Autodesk Inventor part; units mm, degrees
ref_plane "YZ Plane" through (0, 0, 0) normal (1, 0, 0) x (0, 1, 0)
ref_plane "XZ Plane" through (0, 0, 0) normal (0, 1, 0) x (-1, 0, 0)
ref_plane "XY Plane" through (0, 0, 0) normal (0, 0, 1) x (1, 0, 0)
sketch "Sketch13" plane through (0, 0, 0) normal (0, 1, 0) x (-1, 0, 0)
  line L0 (0, 0) -> (112, 0)
  line L1 (112, 0) -> (112, 40)
  line L2 (112, 40) -> (0, 40)
  line L3 (0, 40) -> (0, 0)
  dimension "d51" = 112
  dimension "d52" = 40
extrude "Extrusion11" add sketch "Sketch13" along normal blind 40
sketch "Sketch14" plane through (-112, 0, 40) normal (0, 0, 1) x (1, 0, 0)
  line L0 (0, 0) -> (0, 40)
  arc A0 (88.2072, 0) -> (23.7928, 0) centre (56, 0) ccw
  line L1 (23.7928, 0) -> (88.2072, 0)
  dimension "d88" = 32.2072
extrude "Extrusion12" cut sketch "Sketch14" against normal blind 40
sketch "Sketch15" plane through (0, 0, 0) normal (0, -1, 0) x (1, 0, 0)
  line L0 (-88.2072, 0) -> (-88.2072, 40)
  line L1 (-112, 40) -> (-88.2072, 40)
  line L2 (-112, 0) -> (-112, 40)
  line L3 (-88.2072, 0) -> (-112, 0)
  line L4 (-100.1315, 0) -> (-100.1315, 2.5) construction
  line L5 (-101.9977, 40) -> (-101.9977, 37.5) construction
  line L6 (-112, 20) -> (-109, 20) construction
  line L7 (-88.2072, 20) -> (-94.2072, 20) construction
  line L8 (-109, 37.5) -> (-96, 37.5)
  line L9 (-96, 37.5) -> (-96, 2.5)
  line L10 (-96, 2.5) -> (-109, 2.5)
  line L11 (-109, 2.5) -> (-109, 37.5)
  line L12 (-23.7928, 40) -> (-23.7928, 0)
  line L13 (-23.7928, 40) -> (-23.7928, 0)
  line L14 (0, 0) -> (-23.7928, 0)
  line L15 (0, 40) -> (0, 0)
  line L16 (-23.7928, 40) -> (0, 40)
  line L17 (0, 20) -> (-3, 20) construction
  line L18 (-11.8964, 0) -> (-11.8964, 2.5) construction
  line L19 (-11.8964, 40) -> (-11.8964, 37.5) construction
  line L20 (-23.7928, 20) -> (-17.7928, 20) construction
  line L21 (-16, 37.5) -> (-3, 37.5)
  line L22 (-3, 37.5) -> (-3, 2.5)
  line L23 (-3, 2.5) -> (-16, 2.5)
  line L24 (-16, 2.5) -> (-16, 37.5)
  dimension "d60" = 2.5
  dimension "d62" = 2.5
  dimension "d63" = 3
  dimension "d64" = 6
  dimension "d65" = 3
  dimension "d66" = 2.5
  dimension "d67" = 2.5
  dimension "d68" = 6
extrude "Extrusion13" cut sketch "Sketch15" against normal blind 30 contours L8 L9 L10 L11 | L21 L22 L23 L24
sketch "Sketch16" plane through (0, 30, 0) normal (0, -1, 0) x (1, 0, 0)
  line L0 (-16, 37.5) -> (-3, 37.5)
  line L1 (-16, 2.5) -> (-16, 37.5)
  line L2 (-3, 2.5) -> (-16, 2.5)
  line L3 (-3, 37.5) -> (-3, 2.5)
  circle A0 centre (-102.5, 20) radius 9
  circle A1 centre (-9.5, 20) radius 9
  point P0 (0, 0)
  dimension "d71" = 18
  dimension "d72" = 18
extrude "Extrusion14" add sketch "Sketch16" along normal blind 30 contours A1 L3 L1 | L1 A1 | A1 L3 | A0
sketch "Sketch17" plane through (0, 0, 0) normal (0, -1, 0) x (1, 0, 0)
  arc A0 (-109, 13.7751) -> (-96, 13.7751) centre (-102.5, 20) ccw
  line L0 (-16, 26.2249) -> (-16, 37.5)
  line L1 (-16, 37.5) -> (-3, 37.5)
  line L2 (-3, 37.5) -> (-3, 26.2249)
  arc A1 (-3, 26.2249) -> (-16, 26.2249) centre (-9.5, 20) ccw
  line L3 (-23.7928, 40) -> (-23.7928, 0)
  line L4 (0, 0) -> (-23.7928, 0)
  line L5 (0, 40) -> (0, 0)
  line L6 (-23.7928, 40) -> (0, 40)
  arc A2 (-16, 13.7751) -> (-3, 13.7751) centre (-9.5, 20) ccw
  line L7 (-3, 13.7751) -> (-3, 2.5)
  line L8 (-3, 2.5) -> (-16, 2.5)
  line L9 (-16, 2.5) -> (-16, 13.7751)
  circle A3 centre (-102.5, 20) radius 5.5
  circle A4 centre (-9.5, 20) radius 5.5
  dimension "d75" = 11
  dimension "d76" = 11
extrude "Extrusion15" cut sketch "Sketch17" against normal blind 76.2 contours A3 | A4
sketch "Sketch18" plane through (0, 40, 0) normal (0, 1, 0) x (1, 0, 0)
  circle A0 centre (-102.5, -20) radius 5.5
  circle A1 centre (-9.5, -20) radius 5.5
  circle A2 centre (-102.5, -20) radius 9
  circle A3 centre (-9.5, -20) radius 9
  dimension "d79" = 18
  dimension "d81" = 18
extrude "Extrusion16" cut sketch "Sketch18" against normal blind 8
fillet "Fillet3" radius 3.175 6 edges at (-16, 15, 2.5) (-3, 15, 2.5) (-16, 15, 37.5) (-3, 15, 37.5) (0, 20, 40) (0, 20, 0)
fillet "Fillet4" radius 3.175 6 edges at (-112, 20, 0) (-112, 20, 40) (-109, 15, 37.5) (-109, 15, 2.5) (-96, 15, 2.5) (-96, 15, 37.5)
fillet "Fillet5" radius 1 8 edges at (-0.9299, 40, 39.0701) (0, 40, 20) (-0.9299, 40, 0.9299) (-56, 40, 0) (-111.0701, 40, 0.9299) (-112, 40, 20) (-111.0701, 40, 39.0701) (-56, 40, 40)
equation "\"d62\" = d60"
equation "\"d65\" = d63"
equation "\"d66\" = d60"
equation "\"d67\" = d66"
equation "\"d68\" = d64"
equation "\"d81\" = d79"
properties part number "2.5 CIM mount" material "ABS Plastic"
Input: part model. Units: mm. Frame: model coordinates. A direction names the side the tool comes from. Coordinates: 2 decimals unless noted, no trailing zeros. Loops run counter-clockwise (first coordinate to the right, second up) from the corner with the lowest first, then second, coordinate; pieces in that order, holes last. Notation, with made-up numbers: (-14, 35.5) -> (-4, 35.5) arc R12 cw to (-4, 52.5) -> close; hole circle Ø3 at (-7, 34.25). An arc over 180 degrees is marked (long way). Write each question's results on one line, items separated by ' | '. Start each with the question number.
Q1. Section D-D, the plane x = -56. Return the cut outline in (y, z), plus the area to 3 significant figures.
Q2. Section C-C, the plane y = 25.5. State how many separate pieces and enclosed holes the cut face has, plus the area to 3 significant figures.
Q3. Section A-A, the plane x = -102.5. Return the cut outline in (y, z).
Q4. Pull-direction query (Z, two-part tool) for faces 4 (the cylindrical face through (-55.3, 32.2, 20.3)), 5 (the cylindrical face through (-3.95, 15.21, 36.59)), 6 (the flat face through (-109, 15, 10)), 7 (the flat face through (-57, 37, 40)); classes: released by +Z, released by -Z, zero draft, split by the parting line, or undercut.
Q5. Pin query (flat end, axial travel): pin 1 (8 mm diameter, centred on x = -45.5, z = 16, fed in from -Y); pin 2 (10 mm diameter, centred on x = -65.5, y = 20.5, fed in from -Z); pin 3 (10 mm diameter, centred on x = -44.5, z = 5, fed in from -Y); pin 4 (14.5 mm diameter, centred on x = -102.5, z = 20, fed in from +Y). Return the tip coordinate at first contact, or that it passes through.
Q6. Section B-B, the plane z = 31. Return the cut outline in (x, y).
Q7. Ray query, line 1 (Z direction, x = -9.5, y = 8.5); line 2 (X direction, y = 33.75, z = 20); line 3 (Z direction, x = -9.5, y = 38). Return the intervals inside material, ascending. Write a range as from..to.
Q8. Reachability of faces 1 (the flat face through (-10, 30, 7)), 2 (the cylindrical face through (-0.95, 19.77, 39.09)), 3 (the flat face through (-14, 32, 24)) from +Z, -Z, +X, -X, +Y, -Y: full face, straight path, thin tool, end or side. Return the list, or none.
Found:
1) outline: (32.21, 0) -> (39, 0) arc R1 ccw to (40, 1) -> (40, 39) arc R1 ccw to (39, 40) -> (32.21, 40) -> close | area: 311 mm2
2) separate pieces: 2 | enclosed holes: 6 | area: 2,240 mm2
3) outline: (0, 0) -> (39, 0) arc R1 ccw to (40, 1) -> (40, 11) -> (32, 11) -> (32, 14.5) -> (0, 14.5) -> (0, 11) -> (30, 11) -> (30, 2.5) -> (0, 2.5) -> close; (0, 25.5) -> (32, 25.5) -> (32, 29) -> (40, 29) -> (40, 39) arc R1 ccw to (39, 40) -> (0, 40) -> (0, 37.5) -> (30, 37.5) -> (30, 29) -> (0, 29) -> close
4) face 4: zero draft | face 5: undercut | face 6: undercut | face 7: released by +Z
5) pin 1: y = 28.76 | pin 2: through | pin 3: y = 27.66 | pin 4: y = 32
6) outline: (-112, 0) -> (-109, 0) -> (-109, 30) -> (-96, 30) -> (-96, 0) -> (-88.21, 0) arc R32.21 cw to (-23.79, 0) -> (-16, 0) -> (-16, 30) -> (-3, 30) -> (-3, 0) -> (0, 0) -> (0, 39) arc R1 ccw to (-1, 40) -> (-111, 40) arc R1 ccw to (-112, 39) -> close
7) line 1: 0..2.5, 11..14.5, 25.5..29, 37.5..40 | line 2: -112..-111.5, -93.5..-18.5, -0.5..0 | line 3: 0..11, 29..40
8) face 1: -Y | face 2: +Z, +X, +Y, -Y | face 3: +Y
